Autodesk Inventor part; units mm, degrees
ref_plane "YZ Plane" through (0, 0, 0) normal (1, 0, 0) x (0, 1, 0)
ref_plane "XZ Plane" through (0, 0, 0) normal (0, 1, 0) x (-1, 0, 0)
ref_plane "XY Plane" through (0, 0, 0) normal (0, 0, 1) x (1, 0, 0)
sketch "スケッチ1" plane through (0, 0, 0) normal (1, 0, 0) x (0, 1, 0)
  line L0 (0, 0) -> (46, 0)
  line L1 (46, 0) -> (46, -80)
  line L2 (46, -80) -> (0, -80)
  line L3 (0, -80) -> (0, 0)
  dimension "d0" = 46
  dimension "d1" = 80
extrude "押し出し1" add sketch "スケッチ1" along normal blind 3
sketch "スケッチ2" plane through (3, 0, 0) normal (1, 0, 0) x (0, 0, -1)
  circle A0 centre (40, 23) radius 21
  line L0 (80, 46) -> (0, 46)
  line L1 (0, 46) -> (0, 0)
  dimension "d4" = 42
  dimension "d5" = 23
  dimension "d6" = 40
extrude "押し出し2" cut sketch "スケッチ2" against normal blind 3
sketch "スケッチ3" plane through (3, 0, 0) normal (1, 0, 0) x (0, 0, -1)
  circle A0 centre (72.5, 41) radius 1.6
  line L0 (80, 0) -> (80, 46)
  line L1 (80, 46) -> (0, 46)
  circle A1 centre (72.5, 5) radius 1.6
  line L2 (0, 0) -> (80, 0)
  circle A2 centre (7.5, 41) radius 1.6
  line L3 (0, 46) -> (0, 0)
  circle A3 centre (7.5, 5) radius 1.6
  dimension "d9" = 3.2
  dimension "d10" = 7.5
  dimension "d11" = 5
  dimension "d12" = 3.2
  dimension "d13" = 5
  dimension "d14" = 3.2
  dimension "d15" = 5
  dimension "d16" = 7.5
  dimension "d17" = 3.2
  dimension "d18" = 5
  dimension "d19" = 7.5
  dimension "d20" = 7.5
hole "穴1" at (3, 41, -7.5) at (3, 5, -7.5) at (3, 5, -72.5) at (3, 41, -72.5) direction (-1, 0, 0) diameter 3.2 depth 3
equation "\"BendRadius\" = Thickness"
equation "\"BendReliefWidth\" = Thickness"
equation "\"BendReliefDepth\" = 0.5 * Thickness"
equation "\"CornerReliefSize\" = 4 * Thickness"
equation "\"MinimumRemnant\" = 2 * Thickness"
equation "\"TransitionRadius\" = BendRadius"
equation "\"JacobiRadiusSize\" = BendRadius"
equation "\"GapSize\" = Thickness"
properties part number "nhk30"
Design review of the part built by this model. Coordinates are the model's own, in mm. Give positions to 0.01 mm unless a question says otherwise; leave off trailing zeros. Write each loop counter-clockwise with the first axis right and the second up, starting at its lowest first coordinate (ties: lowest second). Pieces come first, ordered by that corner, then holes. Notation, with made-up numbers: M 39.25,34.25 L 77.25,34.25 A21 ccw 77.25,40.25 Z; hole C 20,86 d6. An arc over 180 degrees is marked long. Return JSON: item names as keys, results as strings. Group by question number.
Item 1: Take a section at A-A (y = 23). Give the boundary of the cut face in (x, z).
Item 2: Take a section at C-C (z = -72.5). Give the boundary of the cut face in (x, y).
Item 3: Take a section at D-D (z = -38.5). Give the boundary of the cut face in (x, y).
Item 4: Wall thickness on line 1 along Y through (x, z) = (1.2, -72.5); line 2 along Z through (x, y) = (2.75, 22.5); line 3 along Z through (x, y) = (2, 41): over which ranges is each line inside the solid? List them lowest first.
Item 5: Take a section at B-B (x = 2.5). Give the boundary of the cut face in (y, z), plus the area to 3 significant figures.
Item 6: The part is to be moulded in two halves that separate along Y. For faces 1 (the flat face through (1, 46, -39)), 2 (the cylindrical face through (1.479, 4.519, -74.026)), 3 (the flat face through (0, 12.46, -21.66)), 4 (the cylindrical face through (1.52, 29.31, -60.03)), say which applies: pulls with the +Y half, pulls with the -Y half, needs draft (parallel to the pull), parting line crosses it, or undercut.
Return value:
{
 "1": {"outline": "M 0,-80 L 3,-80 L 3,-61 L 0,-61 Z; M 0,-19 L 3,-19 L 3,0 L 0,0 Z"},
 "2": {"outline": "M 0,0 L 3,0 L 3,3.4 L 0,3.4 Z; M 0,6.6 L 3,6.6 L 3,39.4 L 0,39.4 Z; M 0,42.6 L 3,42.6 L 3,46 L 0,46 Z"},
 "3": {"outline": "M 0,0 L 3,0 L 3,2.05 L 0,2.05 Z; M 0,43.95 L 3,43.95 L 3,46 L 0,46 Z"},
 "4": {"line 1": "y = 0 to 3.4, 6.6 to 39.4, 42.6 to 46", "line 2": "z = -80 to -60.99, -19.01 to 0", "line 3": "z = -80 to -74.1, -70.9 to -50.82, -29.18 to -9.1, -5.9 to 0"},
 "5": {"outline": "M 0,-80 L 46,-80 L 46,0 L 0,0 Z; hole C 23,-40 d42; hole C 5,-72.5 d3.2; hole C 5,-7.5 d3.2; hole C 41,-72.5 d3.2; hole C 41,-7.5 d3.2", "area": "2,260 mm2"},
 "6": {"face 1": "pulls with the +Y half", "face 2": "undercut", "face 3": "needs draft", "face 4": "undercut"}
}
